Verification items for the finished model (mm, model axes). A direction names the side the tool comes from. Round coordinates to 2 decimals unless told otherwise and drop trailing zeros. Order: outer loops, then holes, each group sorted by start corner. A loop starts at its lowest first (then second) coordinate and runs counter-clockwise, first axis right, second up. Notation, with made-up numbers: (6, -4.5) -> (58, -4.5) arc R24 ccw to (58, 14.5) -> close; hole circle Ø2 at (-19.5, 25). An arc over 180 degrees is marked (long way). Answer in a Markdown table with one row per item. Add a question column.
```python
from build123d import *

# Parameters (mm, degrees)
SKETCH1_W           = 70
SKETCH1_H           = 30
BOSS_EXTRUDE1_DEPTH = 35
CUT_EXTRUDE1_DEPTH  = 20
SKETCH3_W           = 20
SKETCH3_H           = 20
CUT_EXTRUDE2_DEPTH  = 71
SKETCH4_R           = 5
CUT_EXTRUDE3_DEPTH  = 16
SKETCH5_R           = 5
CUT_EXTRUDE4_DEPTH  = 16


with BuildPart() as part:
    # Sketch1 → Boss-Extrude1 (new body)
    with BuildSketch(Plane(origin=(0, 0, 0), x_dir=(1, 0, 0), z_dir=(0, 1, 0))):
        with Locations((35, 15)):
            Rectangle(SKETCH1_W, SKETCH1_H)
    extrude(amount=BOSS_EXTRUDE1_DEPTH)

    # Sketch2 → Cut-Extrude1 (cut)
    with BuildSketch(Plane(origin=(0, 0, -30), x_dir=(-1, 0, 0), z_dir=(0, 0, -1))):
        Polygon((-70, 35), (-70, 10), (-20, 35), align=None)
    extrude(amount=-CUT_EXTRUDE1_DEPTH, mode=Mode.SUBTRACT)

    # Sketch3 → Cut-Extrude2 (cut, through all)
    with BuildSketch(Plane.ZY):
        with Locations((-10, 25)):
            Rectangle(SKETCH3_W, SKETCH3_H)
    extrude(amount=-CUT_EXTRUDE2_DEPTH, mode=Mode.SUBTRACT)

    # Sketch4 → Cut-Extrude3 (cut, through all)
    with BuildSketch(Plane(origin=(0, 15, 0), x_dir=(1, 0, 0), z_dir=(0, 1, 0))):
        with Locations((15, 10)):
            Circle(SKETCH4_R)
    extrude(amount=-CUT_EXTRUDE3_DEPTH, mode=Mode.SUBTRACT)

    # Sketch5 → Cut-Extrude4 (cut, through all)
    with BuildSketch(Plane(origin=(0, 15, 0), x_dir=(1, 0, 0), z_dir=(0, 1, 0))):
        with Locations((45, 10)):
            Circle(SKETCH5_R)
    extrude(amount=-CUT_EXTRUDE4_DEPTH, mode=Mode.SUBTRACT)


solid = part.part
```
1) Cross-section at C-C, the plane z = -7.25. Record the boundary of the cut face in (x, y), and give its area (3 significant figures).
2) Cross-section at A-A, the plane x = 15. Record the boundary of the cut face in (y, z), and give its area (3 significant figures).
3) Thickness scan on L1, parallel to X at y = 9, z = -10; L2, parallel to Z at x = 45, y = 10.75; L3, parallel to Y at x = 36.5, z = -10. Record the ranges inside material, lowest first. Write a range as [from, to].
4) Cross-section at B-B, the plane y = 5.5. Record the boundary of the cut face in (x, z).
5) Depth check by flat-ended pin: P1, Ø4, axis at y = 27, z = -19, coming from the +X side; P2, Ø5, axis at x = 37, z = -17, coming from the +Y side; P3, Ø2, axis at x = 57.5, y = 19.5, coming from the -Z side; P4, Ø1, axis at x = 38, z = -19.5, coming from the -Y side. Enter the tip coordinate at first touch or a pass-through.
6) Cross-section at D-D, the plane x = 45. Record the boundary of the cut face in (y, z), and give its area (3 significant figures).
7) Draft check along X on faces 4 (the face through (0, 13, -18)), 5 (the face through (35, 0, -15)), 6 (the face through (19.77, 7.6, -11.5)), 7 (the face through (70, 6, -15)). Enter one of: +X half, -X half, draft (parallel to the pull), parting line (faces both ways), or undercut.
8) Tool access check on faces 1 (the face through (35, 15, -10)), 2 (the face through (50.906, 19.547, -22.362)), 3 (the face through (27, 13, -30)). Record the directions out of +Z, -Z, +X, -X, +Y, -Y that give a thin tool (end or side, any length) a straight path to the whole face; none if there is none.
Results below:
| question | item | result |
|---|---|---|
| 1 | outline | (0, 0) -> (10.82, 0) -> (10.82, 15) -> (0, 15) -> close; (19.18, 0) -> (40.82, 0) -> (40.82, 15) -> (19.18, 15) -> close; (49.18, 0) -> (70, 0) -> (70, 15) -> (49.18, 15) -> close |
| 1 | area | 799 mm² |
| 2 | outline | (0, -30) -> (35, -30) -> (35, -20) -> (15, -20) -> (15, -15) -> (0, -15) -> close; (0, -5) -> (15, -5) -> (15, 0) -> (0, 0) -> close |
| 2 | area | 500 mm² |
| 3 | L1 | [0, 10], [20, 40], [50, 70] |
| 3 | L2 | [-30, -15], [-5, 0] |
| 3 | L3 | [0, 15] |
| 4 | outline | (0, -30) -> (70, -30) -> (70, 0) -> (0, 0) -> close; hole circle Ø10 at (15, -10); hole circle Ø10 at (45, -10) |
| 5 | P1 | x = 39.46 |
| 5 | P2 | y = 15 |
| 5 | P3 | through |
| 5 | P4 | y = 0 |
| 6 | outline | (0, -30) -> (22.5, -30) -> (22.5, -20) -> (15, -20) -> (15, -15) -> (0, -15) -> close; (0, -5) -> (15, -5) -> (15, 0) -> (0, 0) -> close |
| 6 | area | 375 mm² |
| 7 | face 4 | -X half |
| 7 | face 5 | draft |
| 7 | face 6 | undercut |
| 7 | face 7 | +X half |
| 8 | face 1 | +Z, +X, -X, +Y |
| 8 | face 2 | -Z, +X, +Y |
| 8 | face 3 | -Z, +X, -X, +Y, -Y |
